Work out the finished part from the listing and answer in its coordinate system (mm). A direction names the side the tool comes from. Coordinates: 2 decimals unless noted, no trailing zeros. Order: outer loops, then holes, each group sorted by start corner. A loop starts at its lowest first (then second) coordinate and runs counter-clockwise, first axis right, second up. Notation, with made-up numbers: M 65.5,5.25 L 96.5,5.25 A17 cw 96.5,23.25 Z; hole C 7.5,62 d1. An arc over 180 degrees is marked long. Use a Markdown table: item, result.
from build123d import *

# Parameters (mm, degrees)
SKETCH_1_W      = 36
SKETCH_1_H      = 14
SKETCH_1_R      = 1.368610336
SKETCH_1_R_2    = 1.290695583
EXTRUDE_1_DEPTH = 5
SKETCH_2_W      = 22
SKETCH_2_H      = 14
EXTRUDE_2_DEPTH = 6
SKETCH_3_W      = 22
SKETCH_3_H      = 14
SKETCH_3_W_2    = 14.5
SKETCH_3_H_2    = 6
EXTRUDE_3_DEPTH = 4
FILLET_1_R      = 3
FILLET_2_R      = 2
FILLET_3_R      = 2
SKETCH_4_W      = 20
SKETCH_4_H      = 12
EXTRUDE_4_DEPTH = 5
FILLET_4_R      = 1


with BuildPart() as part:
    # Эскиз1 → Бобышка-Вытянуть1 (new body)
    with BuildSketch(Plane.XY):
        with Locations((8, -4)):
            Rectangle(SKETCH_1_W, SKETCH_1_H)
        with Locations((-7, -4)):
            Circle(SKETCH_1_R, mode=Mode.SUBTRACT)
        with Locations((23, -4)):
            Circle(SKETCH_1_R_2, mode=Mode.SUBTRACT)
        Polygon((13.7, 0), (16.5, -2.8), (16.5, -5.2), (13.7, -8), (0, -8), (0, 0), align=None, mode=Mode.SUBTRACT)
    extrude(amount=EXTRUDE_1_DEPTH)

    # Эскиз2 → Бобышка-Вытянуть2 (add)
    with BuildSketch(Plane(origin=(0, 0, 0), x_dir=(-1, 0, 0), z_dir=(0, 0, -1))):
        with Locations((-8, -4)):
            Rectangle(SKETCH_2_W, SKETCH_2_H)
        Polygon((-16.5, -2.8), (-13.7, 0), (0, 0), (0, -8), (-13.7, -8), (-16.5, -5.2), align=None, mode=Mode.SUBTRACT)
    extrude(amount=EXTRUDE_2_DEPTH)

    # Эскиз3 → Бобышка-Вытянуть3 (add)
    with BuildSketch(Plane(origin=(0, 0, -6), x_dir=(-1, 0, 0), z_dir=(0, 0, -1))):
        with Locations((-8, -4)):
            Rectangle(SKETCH_3_W, SKETCH_3_H)
        with Locations((-8.25, -4)):
            Rectangle(SKETCH_3_W_2, SKETCH_3_H_2, mode=Mode.SUBTRACT)
    extrude(amount=EXTRUDE_3_DEPTH)

    # Скругление1
    fillet_1_edges = [part.edges().sort_by_distance(p)[0] for p in [
        (-10, 3, 2.5),
        (26, 3, 2.5),
        (26, -11, 2.5),
        (-10, -11, 2.5),
    ]]
    fillet(fillet_1_edges, radius=FILLET_1_R)

    # Скругление2
    # the kernel refuses this fillet: 2 mm, written as the material it adds along each edge
    with BuildSketch(Plane(origin=(15.5, -7, -6), x_dir=(0, 1, 0), z_dir=(0, 0, -1)), Plane(origin=(1, -7, -6), x_dir=(1, 0, 0), z_dir=(0, 0, -1)), Plane(origin=(1, -1, -6), x_dir=(0, -1, 0), z_dir=(0, 0, -1))) as fillet_2_piece_1:
        with BuildLine():
            CenterArc((FILLET_2_R, -FILLET_2_R), FILLET_2_R, 90, 90)
            Line((0, -FILLET_2_R), (0, 0))
            Line((0, 0), (FILLET_2_R, 0))
        make_face()
    extrude(amount=4)
    with BuildSketch(Plane(origin=(15.5, -1, -6), x_dir=(0, -1, 0), z_dir=(0, 0, -1))) as fillet_2_piece_2:
        with BuildLine():
            CenterArc((FILLET_2_R, FILLET_2_R), FILLET_2_R, 180, 90)
            Line((0, FILLET_2_R), (0, 0))
            Line((0, 0), (FILLET_2_R, 0))
        make_face()
    extrude(amount=4)
    # the kernel refuses this fillet: 2 mm, written as the material it takes off along each edge
    with BuildSketch(Plane(origin=(19, 3, 0), x_dir=(-1, 0, 0), z_dir=(0, 0, -1)), Plane(origin=(-3, 3, -15), x_dir=(1, 0, 0), z_dir=(0, 0, 1))) as fillet_2_2_piece_1:
        with BuildLine():
            CenterArc((FILLET_2_R, -FILLET_2_R), FILLET_2_R, 90, 90)
            Line((0, -FILLET_2_R), (0, 0))
            Line((0, 0), (FILLET_2_R, 0))
        make_face()
    extrude(amount=15, mode=Mode.SUBTRACT)
    with BuildSketch(Plane(origin=(19, -11, 0), x_dir=(-1, 0, 0), z_dir=(0, 0, -1)), Plane(origin=(-3, -11, -15), x_dir=(1, 0, 0), z_dir=(0, 0, 1))) as fillet_2_2_piece_2:
        with BuildLine():
            CenterArc((FILLET_2_R, FILLET_2_R), FILLET_2_R, 180, 90)
            Line((0, FILLET_2_R), (0, 0))
            Line((0, 0), (FILLET_2_R, 0))
        make_face()
    extrude(amount=15, mode=Mode.SUBTRACT)

    # Скругление3
    # the kernel refuses this fillet: 2 mm, written as the material it takes off along each edge
    with BuildSketch(Plane(origin=(13.5, -1, -10), x_dir=(0, 1, 0), z_dir=(-1, 0, 0)), Plane(origin=(3, -7, -10), x_dir=(0, -1, 0), z_dir=(1, 0, 0))) as fillet_3_piece_1:
        with BuildLine():
            CenterArc((FILLET_3_R, -FILLET_3_R), FILLET_3_R, 90, 90)
            Line((0, -FILLET_3_R), (0, 0))
            Line((0, 0), (FILLET_3_R, 0))
        make_face()
    extrude(amount=10.5, mode=Mode.SUBTRACT)
    with BuildSketch(Plane(origin=(15.5, -5, -10), x_dir=(1, 0, 0), z_dir=(0, 1, 0)), Plane(origin=(1, -3, -10), x_dir=(-1, 0, 0), z_dir=(0, -1, 0))) as fillet_3_piece_2:
        with BuildLine():
            CenterArc((FILLET_3_R, -FILLET_3_R), FILLET_3_R, 90, 90)
            Line((0, -FILLET_3_R), (0, 0))
            Line((0, 0), (FILLET_3_R, 0))
        make_face()
    extrude(amount=2, mode=Mode.SUBTRACT)
    with BuildSketch(Plane(origin=(-3, 1, -10), x_dir=(1, 0, 0), z_dir=(0, -1, 0)), Plane(origin=(19, -9, -10), x_dir=(-1, 0, 0), z_dir=(0, 1, 0))) as fillet_3_piece_3:
        with BuildLine():
            CenterArc((FILLET_3_R, FILLET_3_R), FILLET_3_R, 180, 90)
            Line((0, FILLET_3_R), (0, 0))
            Line((0, 0), (FILLET_3_R, 0))
        make_face()
    extrude(amount=10, mode=Mode.SUBTRACT)
    with BuildSketch(Plane(origin=(-1, -11, -10), x_dir=(0, 1, 0), z_dir=(1, 0, 0)), Plane(origin=(17, 3, -10), x_dir=(0, -1, 0), z_dir=(-1, 0, 0))) as fillet_3_piece_4:
        with BuildLine():
            CenterArc((FILLET_3_R, FILLET_3_R), FILLET_3_R, 180, 90)
            Line((0, FILLET_3_R), (0, 0))
            Line((0, 0), (FILLET_3_R, 0))
        make_face()
    extrude(amount=18, mode=Mode.SUBTRACT)
    with BuildSketch(Plane(origin=(17, 1, -10), x_dir=(1, 0, 0), z_dir=(0, -1, 0))) as fillet_3_piece_5:
        with BuildLine():
            CenterArc((2 - FILLET_3_R, FILLET_3_R), FILLET_3_R, 270, 90)
            Line((2, FILLET_3_R), (2, 0))
            Line((2, 0), (2 - FILLET_3_R, 0))
        make_face()
    revolve(axis=Axis((17, 1, -10), (0, 0, 1)), revolution_arc=90, mode=Mode.SUBTRACT)
    with BuildSketch(Plane(origin=(17, -9, -10), x_dir=(0, -1, 0), z_dir=(-1, 0, 0))) as fillet_3_piece_6:
        with BuildLine():
            CenterArc((2 - FILLET_3_R, FILLET_3_R), FILLET_3_R, 270, 90)
            Line((2, FILLET_3_R), (2, 0))
            Line((2, 0), (2 - FILLET_3_R, 0))
        make_face()
    revolve(axis=Axis((17, -9, -10), (0, 0, 1)), revolution_arc=90, mode=Mode.SUBTRACT)
    with BuildSketch(Plane(origin=(-1, 1, -10), x_dir=(-1, 0, 0), z_dir=(0, -1, 0))) as fillet_3_piece_7:
        with BuildLine():
            CenterArc((2 - FILLET_3_R, -FILLET_3_R), FILLET_3_R, 0, 90)
            Line((2, -FILLET_3_R), (2, 0))
            Line((2, 0), (2 - FILLET_3_R, 0))
        make_face()
    revolve(axis=Axis((-1, 1, -10), (0, 0, -1)), revolution_arc=90, mode=Mode.SUBTRACT)
    with BuildSketch(Plane(origin=(-1, -9, -10), x_dir=(0, -1, 0), z_dir=(1, 0, 0))) as fillet_3_piece_8:
        with BuildLine():
            CenterArc((2 - FILLET_3_R, -FILLET_3_R), FILLET_3_R, 0, 90)
            Line((2, -FILLET_3_R), (2, 0))
            Line((2, 0), (2 - FILLET_3_R, 0))
        make_face()
    revolve(axis=Axis((-1, -9, -10), (0, 0, -1)), revolution_arc=90, mode=Mode.SUBTRACT)
    with BuildSketch(Plane(origin=(13.5, -3, -10), x_dir=(0, 1, 0), z_dir=(-1, 0, 0))) as fillet_3_piece_9:
        with BuildLine():
            CenterArc((2 + FILLET_3_R, -FILLET_3_R), FILLET_3_R, 90, 90)
            Line((2 + FILLET_3_R, 0), (2, 0))
            Line((2, 0), (2, -FILLET_3_R))
        make_face()
    revolve(axis=Axis((13.5, -3, -10), (0, 0, -1)), revolution_arc=90, mode=Mode.SUBTRACT)
    with BuildSketch(Plane(origin=(13.5, -5, -10), x_dir=(1, 0, 0), z_dir=(0, 1, 0))) as fillet_3_piece_10:
        with BuildLine():
            CenterArc((2 + FILLET_3_R, -FILLET_3_R), FILLET_3_R, 90, 90)
            Line((2, -FILLET_3_R), (2, 0))
            Line((2, 0), (2 + FILLET_3_R, 0))
        make_face()
    revolve(axis=Axis((13.5, -5, -10), (0, 0, -1)), revolution_arc=90, mode=Mode.SUBTRACT)
    with BuildSketch(Plane(origin=(3, -5, -10), x_dir=(0, -1, 0), z_dir=(1, 0, 0))) as fillet_3_piece_11:
        with BuildLine():
            CenterArc((2 + FILLET_3_R, -FILLET_3_R), FILLET_3_R, 90, 90)
            Line((2, -FILLET_3_R), (2, 0))
            Line((2, 0), (2 + FILLET_3_R, 0))
        make_face()
    revolve(axis=Axis((3, -5, -10), (0, 0, -1)), revolution_arc=90, mode=Mode.SUBTRACT)
    with BuildSketch(Plane(origin=(3, -3, -10), x_dir=(-1, 0, 0), z_dir=(0, -1, 0))) as fillet_3_piece_12:
        with BuildLine():
            CenterArc((2 + FILLET_3_R, -FILLET_3_R), FILLET_3_R, 90, 90)
            Line((2, -FILLET_3_R), (2, 0))
            Line((2, 0), (2 + FILLET_3_R, 0))
        make_face()
    revolve(axis=Axis((3, -3, -10), (0, 0, -1)), revolution_arc=90, mode=Mode.SUBTRACT)

    # Эскиз4 → Бобышка-Вытянуть4 (add)
    with BuildSketch(Plane.XY.offset(5)):
        with Locations((8, -4)):
            Rectangle(SKETCH_4_W, SKETCH_4_H)
        Polygon((0, 0), (13.7, 0), (16.5, -2.8), (16.5, -5.2), (13.7, -8), (0, -8), align=None, mode=Mode.SUBTRACT)
    extrude(amount=EXTRUDE_4_DEPTH)

    # Скругление4
    fillet_4_edges = [part.edges().sort_by_distance(p)[0] for p in [
        (-2, 2, 7.5),
        (-2, -10, 7.5),
        (18, -10, 7.5),
        (18, 2, 7.5),
    ]]
    fillet(fillet_4_edges, radius=FILLET_4_R)


solid = part.part
1. Section C-C on x = 13 is taken. Determine the outline of the cut face in (y, z).
Answers below:
| item | result |
|---|---|
| outline | M -11,-8 A2 ccw -7,-8 L -7,-6 L -8,-6 L -8,10 L -10,10 L -10,5 L -11,5 Z; M -1,-8 A2 ccw 3,-8 L 3,5 L 2,5 L 2,10 L 0,10 L 0,-6 L -1,-6 Z |
2. For faces 4 (the face through (6.4, -7.3, -6)), 5 (the face through (8, -7, -7)), 6 (the face through (-1.715, 1.699, 7.535)), determine the directions among +Z, -Z, +X, -X, +Y, -Y from which every point of the face is accessible in a straight line to the end or side of a thin tool.
Answers below:
| item | result |
|---|---|
| face 4 | +Z |
| face 5 | +Z, -Z |
| face 6 | +Z, -X, +Y |
3. Section A-A on y = -4 is taken. Give the number of separate pieces and of enclosed holes in the cut face, then the cut area to 3 significant figures.
Answers below:
| item | result |
|---|---|
| separate pieces | 4 |
| enclosed holes | 0 |
| area | 148 mm² |
4. Section D-D on z = -7.5 is taken. Determine the outline of the cut face in (x, y).
Answers below:
| item | result |
|---|---|
| outline | M -3,-9 A2 ccw -1,-11 L 17,-11 A2 ccw 19,-9 L 19,1 A2 ccw 17,3 L -1,3 A2 ccw -3,1 Z; hole M 1,-5 A2 ccw 3,-7 L 13.5,-7 A2 ccw 15.5,-5 L 15.5,-3 A2 ccw 13.5,-1 L 3,-1 A2 ccw 1,-3 Z |
5. Flat-ended cylindrical pins translate along their axes: P1, Ø2, axis at y = -9.5, z = -3, coming from the +X side; P2, Ø2.5, axis at x = 9, z = 8.5, coming from the -Y side; P3, Ø2, axis at x = -7, y = -4, coming from the +Z side; P4, Ø2.5, axis at y = -5, z = 7.5, coming from the +X side. Find the tip coordinate at first contact, or state that the pin passes through.
Answers below:
| item | result |
|---|---|
| P1 | x = 19 |
| P2 | y = -10 |
| P3 | through |
| P4 | x = 18 |
6. For a pull along X with two mould halves and no side action, classify faces 1 (the face through (21, -4, 0)), 2 (the face through (17.715, -9.699, 7.535)), 3 (the face through (15.5, -4, -7)) as +X half, -X half, draft (parallel to the pull), parting line (faces both ways), or undercut.
Answers below:
| item | result |
|---|---|
| face 1 | draft |
| face 2 | +X half |
| face 3 | undercut |
7. Section B-B on z = 1.5 is taken. Determine the outline of the cut face in (x, y), then the cut area to 3 significant figures.
Answers below:
| item | result |
|---|---|
| outline | M -10,-8 A3 ccw -7,-11 L 23,-11 A3 ccw 26,-8 L 26,0 A3 ccw 23,3 L -7,3 A3 ccw -10,0 Z; hole C -7,-4 d2.74; hole M 0,-8 L 13.7,-8 L 16.5,-5.2 L 16.5,-2.8 L 13.7,0 L 0,0 Z; hole C 23,-4 d2.58 |
| area | 361 mm² |
8. Find the intervals of material crossed by probe 1 along Y at (x, z) = (23, 3.15); probe 2 along Y at (x, z) = (0.5, 2); probe 3 along X at (y, z) = (-0.25, 1), in increasing order.
Answers below:
| item | result |
|---|---|
| probe 1 | -11 to -5.29, -2.71 to 3 |
| probe 2 | -11 to -8, 0 to 3 |
| probe 3 | -10 to 0, 13.95 to 26 |
